The model under review builds one solid part; all positions refer to its coordinate system, in mm. Round coordinates to 2 decimals unless told otherwise and drop trailing zeros. Write each loop counter-clockwise with the first axis right and the second up, starting at its lowest first coordinate (ties: lowest second). Pieces come first, ordered by that corner, then holes. Notation, with made-up numbers: (89, 35) -> (99, 35) arc R18 cw to (99, 55) -> close; hole circle Ø4 at (41.25, -17.5). An arc over 180 degrees is marked (long way). Answer as a JSON object with one key per item and string values. Group by question number.
1) Insertion check: pin 1 Ø17 at (x, y) = (-38.5, 387.5) entering from +Z; pin 2 Ø20.5 at (x, y) = (5.5, -2) entering from -Z; pin 3 Ø8 at (x, y) = (-13.5, -925.5) entering from +Z; pin 4 Ø1 at (x, y) = (22.5, 263) entering from +Z. Each pin has a flat end and moves straight along its axis. Give the tip position at first contact, or say it passes through.
2) We need section A-A, the plane z = -21. Write out the cut boundary in (x, y), then the cut area to 3 significant figures.
3) We need section B-B, the plane y = 1001. Write out the cut boundary in (x, z).
4) To check wall thickness, follow probe 1 along Y at (x, z) = (0, -0.75); probe 2 along X at (y, z) = (106.5, -10); probe 3 along X at (y, z) = (1201.5, -1.1). State the ranges of each line that lie inside material, in increasing order. Write a range as [from, to].
from build123d import *

# Parameters (mm, degrees)
SKETCH1_W                      = 50
SKETCH1_H                      = 2443
BASE_FLANGE1_DEPTH             = 2
EDGE_FLANGE1_STRIP_W           = 13
EDGE_FLANGE1_STRIP_H           = 2
EDGE_FLANGE1_STRIP_CUT_DEPTH   = 2443
EDGE_FLANGE1_STRIP_2_W         = 13
EDGE_FLANGE1_STRIP_2_H         = 2
EDGE_FLANGE1_STRIP_CUT_2_DEPTH = 2443
EDGE_FLANGE1_DEPTH             = 2443
EDGE_FLANGE1_BEND_DEPTH        = 2443
EDGE_FLANGE2_STRIP_W           = 13
EDGE_FLANGE2_STRIP_H           = 2
EDGE_FLANGE2_STRIP_CUT_DEPTH   = 2443
EDGE_FLANGE2_STRIP_2_W         = 13
EDGE_FLANGE2_STRIP_2_H         = 2
EDGE_FLANGE2_STRIP_CUT_2_DEPTH = 2443
EDGE_FLANGE2_DEPTH             = 2443
EDGE_FLANGE2_BEND_DEPTH        = 2443
SKETCH18_R                     = 5.5
CUT_EXTRUDE1_DEPTH             = 10


# Sheet-metal steps are written as plain solids
with BuildPart() as part:
    # Sketch1 → Base-Flange1 (new body)
    with BuildSketch(Plane.XY):
        Rectangle(SKETCH1_W, SKETCH1_H)
    extrude(amount=-BASE_FLANGE1_DEPTH)

    # Edge-Flange1 strip (across the edge) → Edge-Flange1 strip cut (cut)
    with BuildSketch(Plane(origin=(25, 1221.5, -2), x_dir=(-1, 0, 0), z_dir=(0, -1, 0))):
        with Locations((-2, -1)):
            Rectangle(EDGE_FLANGE1_STRIP_W, EDGE_FLANGE1_STRIP_H)
    extrude(amount=EDGE_FLANGE1_STRIP_CUT_DEPTH, mode=Mode.SUBTRACT)

    # Edge-Flange1 strip 2 (across the edge) → Edge-Flange1 strip cut 2 (cut)
    with BuildSketch(Plane(origin=(-25, -1221.5, -2), x_dir=(1, 0, 0), z_dir=(0, 1, 0))):
        with Locations((-2, -1)):
            Rectangle(EDGE_FLANGE1_STRIP_2_W, EDGE_FLANGE1_STRIP_2_H)
    extrude(amount=EDGE_FLANGE1_STRIP_CUT_2_DEPTH, mode=Mode.SUBTRACT)

    # Edge-Flange1 section (across the edge) → Edge-Flange1 (add)
    with BuildSketch(Plane(origin=(25, 1221.5, -2), x_dir=(-1, 0, 0), z_dir=(0, -1, 0))):
        with BuildLine():
            Line((0, 2.5), (0, 28))
            Line((0, 28), (2, 28))
            Line((2, 28), (2, 2.5))
            ThreePointArc((2, 2.5), (2.732233047, 0.732233047), (4.5, 0))
            Line((4.5, 0), (4.5, -2))
            ThreePointArc((4.5, -2), (1.318019485, -0.681980515), (0, 2.5))
        make_face()
    extrude(amount=EDGE_FLANGE1_DEPTH)

    # Edge-Flange1 section 2 (across the edge) → Edge-Flange1 bend (add)
    with BuildSketch(Plane(origin=(-25, -1221.5, -2), x_dir=(1, 0, 0), z_dir=(0, 1, 0))):
        with BuildLine():
            Line((0, 2.5), (0, 28))
            Line((0, 28), (2, 28))
            Line((2, 28), (2, 2.5))
            ThreePointArc((2, 2.5), (2.732233047, 0.732233047), (4.5, 0))
            Line((4.5, 0), (4.5, -2))
            ThreePointArc((4.5, -2), (1.318019485, -0.681980515), (0, 2.5))
        make_face()
    extrude(amount=EDGE_FLANGE1_BEND_DEPTH)

    # Edge-Flange2 strip (across the edge) → Edge-Flange2 strip cut (cut)
    with BuildSketch(Plane(origin=(-25, 1221.5, -30), x_dir=(0, 0, 1), z_dir=(0, -1, 0))):
        with Locations((-2, -1)):
            Rectangle(EDGE_FLANGE2_STRIP_W, EDGE_FLANGE2_STRIP_H)
    extrude(amount=EDGE_FLANGE2_STRIP_CUT_DEPTH, mode=Mode.SUBTRACT)

    # Edge-Flange2 strip 2 (across the edge) → Edge-Flange2 strip cut 2 (cut)
    with BuildSketch(Plane(origin=(25, -1221.5, -30), x_dir=(0, 0, 1), z_dir=(0, 1, 0))):
        with Locations((-2, -1)):
            Rectangle(EDGE_FLANGE2_STRIP_2_W, EDGE_FLANGE2_STRIP_2_H)
    extrude(amount=EDGE_FLANGE2_STRIP_CUT_2_DEPTH, mode=Mode.SUBTRACT)

    # Edge-Flange2 section (across the edge) → Edge-Flange2 (add)
    with BuildSketch(Plane(origin=(-25, 1221.5, -30), x_dir=(0, 0, 1), z_dir=(0, -1, 0))):
        with BuildLine():
            Line((0, 2.5), (0, 18))
            Line((0, 18), (2, 18))
            Line((2, 18), (2, 2.5))
            ThreePointArc((2, 2.5), (2.732233047, 0.732233047), (4.5, 0))
            Line((4.5, 0), (4.5, -2))
            ThreePointArc((4.5, -2), (1.318019485, -0.681980515), (0, 2.5))
        make_face()
    extrude(amount=EDGE_FLANGE2_DEPTH)

    # Edge-Flange2 section 2 (across the edge) → Edge-Flange2 bend (add)
    with BuildSketch(Plane(origin=(25, -1221.5, -30), x_dir=(0, 0, 1), z_dir=(0, 1, 0))):
        with BuildLine():
            Line((0, 2.5), (0, 18))
            Line((0, 18), (2, 18))
            Line((2, 18), (2, 2.5))
            ThreePointArc((2, 2.5), (2.732233047, 0.732233047), (4.5, 0))
            Line((4.5, 0), (4.5, -2))
            ThreePointArc((4.5, -2), (1.318019485, -0.681980515), (0, 2.5))
        make_face()
    extrude(amount=EDGE_FLANGE2_BEND_DEPTH)

    # Sketch18 → Cut-Extrude1 (cut)
    with BuildSketch(Plane(origin=(0, 0, -2), x_dir=(-1, 0, 0), z_dir=(0, 0, -1))):
        with Locations((0, 1201.5)):
            Circle(SKETCH18_R)
    cut_extrude1 = extrude(amount=-CUT_EXTRUDE1_DEPTH, mode=Mode.SUBTRACT)

    # Mirror1: Cut-Extrude1 across plane
    add(cut_extrude1.mirror(Plane.ZX), mode=Mode.SUBTRACT)


solid = part.part
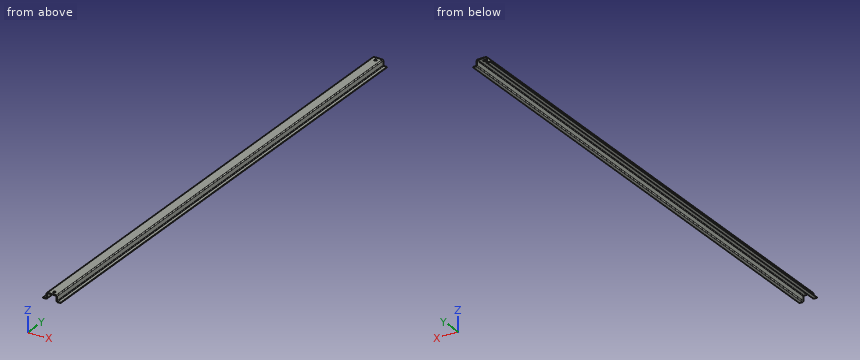
Here are the results:
{
 "1": {"pin 1": "stops at z = -28", "pin 2": "stops at z = -2", "pin 3": "stops at z = 0", "pin 4": "stops at z = -0.26"},
 "2": {"outline": "(-25, -1221.5) -> (-23, -1221.5) -> (-23, 1221.5) -> (-25, 1221.5) -> close; (23, -1221.5) -> (25, -1221.5) -> (25, 1221.5) -> (23, 1221.5) -> close", "area": "9,770 mm^2"},
 "3": {"outline": "(-43, -30) -> (-27.5, -30) arc R4.5 ccw to (-23, -25.5) -> (-23, -4.5) arc R2.5 cw to (-20.5, -2) -> (20.5, -2) arc R2.5 cw to (23, -4.5) -> (23, -25.5) arc R4.5 ccw to (27.5, -30) -> (43, -30) -> (43, -28) -> (27.5, -28) arc R2.5 cw to (25, -25.5) -> (25, -4.5) arc R4.5 ccw to (20.5, 0) -> (-20.5, 0) arc R4.5 ccw to (-25, -4.5) -> (-25, -25.5) arc R2.5 cw to (-27.5, -28) -> (-43, -28) -> close"},
 "4": {"probe 1": "y = [-1221.5, -1207], [-1196, 1196], [1207, 1221.5]", "probe 2": "x = [-25, -23], [23, 25]", "probe 3": "x = [-23.45, -5.5], [5.5, 23.45]"}
}
